Read the model definition and answer for the solid it produces. Units are mm, in the model's axes. A direction names the side the tool comes from. Give positions to 0.01 mm unless a question says otherwise; leave off trailing zeros. Write each loop counter-clockwise with the first axis right and the second up, starting at its lowest first coordinate (ties: lowest second). Pieces come first, ordered by that corner, then holes. Notation, with made-up numbers: (15.25, -0.75) -> (64.25, -0.75) arc R13 cw to (64.25, 18.25) -> close; hole circle Ø9 at (15.25, -25.5). An arc over 180 degrees is marked (long way). Put each result on its own line as item: value. Start each with the question number.
from build123d import *

# Parameters (mm, degrees)
F0_R     = 10
F1_DEPTH = 6.5
F2_DEPTH = 2
F3_SIZE2 = 0.5773502692
F3_SIZE  = 1


with BuildPart() as f1:
    # F0 (on Top) → F1 (new body)
    with BuildSketch(Plane.XY):
        Circle(F0_R)
        Polygon((-5.55625, -3.2079024332), (-5.55625, 3.2079024332), (0, 6.4158048664), (5.55625, 3.2079024332), (5.55625, -3.2079024332), (0, -6.4158048664), align=None, mode=Mode.SUBTRACT)
    extrude(amount=F1_DEPTH)

    # F0 (on Top) → F2 (join)
    with BuildSketch(Plane.XY):
        Polygon((0, 6.4158048664), (-5.55625, 3.2079024332), (-5.55625, -3.2079024332), (0, -6.4158048664), (5.55625, -3.2079024332), (5.55625, 3.2079024332), align=None)
    extrude(amount=F2_DEPTH)

    # F3
    f3_edges = [f1.edges().sort_by_distance(p)[0] for p in [
        (-10, 0, 0),
    ]]
    f3_side = f1.faces().sort_by_distance((-10, 0, 3.25))[0]
    chamfer(f3_edges, length=F3_SIZE, length2=F3_SIZE2, reference=f3_side)


solid = f1.part
1) Straight lines are drawn through the part: line 1 (Z direction, x = 0.25, y = -3.25); line 2 (X direction, y = -3, z = 4.75); line 3 (Y direction, x = -1.25, z = 6). For each, find the intervals that lie inside material, in ascending order. Write a range as [from, to].
2) For faces 1 (the face through (2.8, -4.8, 4.2)), 2 (the face through (4.3, -4.3, 6.5)), determine the directions among +Z, -Z, +X, -X, +Y, -Y from which every point of the face is accessible in a straight line to the end or side of a thin tool.
3) A cutting plane is placed at A-A on z = 6. Give the vertices of the cut face in (x, y), and give its area (3 significant figures).
4) For a pull along X with two mould halves and no side action, classify faces 3 (the face through (-2.8, 4.8, 4.2)), 4 (the face through (-2.17, -9.76, 3.71)), 5 (the face through (0, 0, 0)) as pulls with the +X half, pulls with the -X half, needs draft (parallel to the pull), parting line crosses it, or undercut.
5) A cutting plane is placed at B-B on y = 0. Give the vertices of the cut face in (x, z).
6) Each of these flat-tipped pins is pushed along its axis until it touches: pin 1 Ø1.5 at (y, z) = (2, 2.5) entering from -X; pin 2 Ø1.5 at (y, z) = (6.5, 5.5) entering from -X; pin 3 Ø1 at (y, z) = (-2, 1.5) entering from +X; pin 4 Ø6 at (x, y) = (5.5, -1) entering from -Z. Where does it stop, or does it pass through?
7) A cutting plane is placed at C-C on z = 1.5. Give the vertices of the cut face in (x, y).
Results found:
1. line 1: z = [0, 2]
1. line 2: x = [-9.54, -5.56], [5.56, 9.54]
1. line 3: y = [-9.92, -5.69], [5.69, 9.92]
2. face 1: +Z
2. face 2: +Z, +X, -X, +Y, -Y
3. outline: circle Ø20 at (0, 0); hole (-5.56, -3.21) -> (0, -6.42) -> (5.56, -3.21) -> (5.56, 3.21) -> (0, 6.42) -> (-5.56, 3.21) -> close
3. area: 207 mm²
4. face 3: undercut
4. face 4: parting line crosses it
4. face 5: needs draft
5. outline: (-10, 1) -> (-9.42, 0) -> (9.42, 0) -> (10, 1) -> (10, 6.5) -> (5.56, 6.5) -> (5.56, 2) -> (-5.56, 2) -> (-5.56, 6.5) -> (-10, 6.5) -> close
6. pin 1: stops at x = -9.92
6. pin 2: stops at x = -8.18
6. pin 3: stops at x = 9.89
6. pin 4: stops at z = 0
7. outline: circle Ø20 at (0, 0)
